from build123d import *

# Parameters (mm, degrees)
SKETCH1_W               = 45
SKETCH1_H               = 67.7
BOSS_EXTRUDE1_DEPTH     = 1.5
CUT_EXTRUDE1_DEPTH      = 41.67336352
CUT_EXTRUDE1_DEPTH_BACK = 41.67336352
SKETCH2_W               = 15
SKETCH2_H               = 3
CUT_EXTRUDE2_DEPTH      = 41.67336352
CUT_EXTRUDE2_DEPTH_BACK = 41.67336352
SKETCH3_R               = 1.5
CUT_EXTRUDE3_DEPTH      = 41.67336352
CUT_EXTRUDE3_DEPTH_BACK = 41.67336352


with BuildPart() as part:
    # Sketch1 → Boss-Extrude1 (new, symmetric)
    with BuildSketch(Plane(origin=(0, 0, 0), x_dir=(1, 0, 0), z_dir=(0, 1, 0))):
        Rectangle(SKETCH1_W, SKETCH1_H)
    extrude(amount=BOSS_EXTRUDE1_DEPTH, both=True)

    # Sketch2 → Cut-Extrude1 (cut, two sides: drawn at the far end of the back side and taken through both)
    with BuildSketch(Plane(origin=(0, 0, 0), x_dir=(1, 0, 0), z_dir=(0, 1, 0)).offset(-CUT_EXTRUDE1_DEPTH_BACK)):
        with Locations((0, -32.35)):
            Rectangle(SKETCH2_W, SKETCH2_H)
        with Locations((0, 32.35)):
            Rectangle(SKETCH2_W, SKETCH2_H)
    extrude(amount=CUT_EXTRUDE1_DEPTH + CUT_EXTRUDE1_DEPTH_BACK, mode=Mode.SUBTRACT)

    # Sketch3 → Cut-Extrude2 (cut, two sides: drawn at the far end of the back side and taken through both)
    with BuildSketch(Plane(origin=(0, 0, 0), x_dir=(1, 0, 0), z_dir=(0, 1, 0)).offset(-CUT_EXTRUDE2_DEPTH_BACK)):
        with Locations(Location((-6.717514421, -17.217514421, 0), (0, 0, 270))):
            Circle(SKETCH3_R)
        with Locations(Location((-6.717514421, 17.217514421, 0), (0, 0, 90))):
            Circle(SKETCH3_R)
        with BuildLine():
            Line((0.072542026, 12.729181386), (-2.119583462, 14.921306874))
            ThreePointArc((-2.119583462, 14.921306874), (-3.083402548, 20.851626294), (-9.013721969, 21.815445381))
            Line((-9.013721969, 21.815445381), (-11.205847457, 24.007570869))
            ThreePointArc((-11.205847457, 24.007570869), (-0.962082205, 22.972946638), (0.072542026, 12.729181386))
        make_face()
        with BuildLine():
            Line((-2.229181386, 10.427457974), (-4.421306874, 12.619583462))
            ThreePointArc((-4.421306874, 12.619583462), (-10.351626294, 13.583402548), (-11.315445381, 19.513721969))
            Line((-11.315445381, 19.513721969), (-13.507570869, 21.705847457))
            ThreePointArc((-13.507570869, 21.705847457), (-12.472946638, 11.462082205), (-2.229181386, 10.427457974))
        make_face()
        with BuildLine():
            Line((0.072542026, -12.729181386), (-2.119583462, -14.921306874))
            ThreePointArc((-2.119583462, -14.921306874), (-3.083402548, -20.851626294), (-9.013721969, -21.815445381))
            Line((-9.013721969, -21.815445381), (-11.205847457, -24.007570869))
            ThreePointArc((-11.205847457, -24.007570869), (-0.962082205, -22.972946638), (0.072542026, -12.729181386))
        make_face()
        with BuildLine():
            Line((-2.229181386, -10.427457974), (-4.421306874, -12.619583462))
            ThreePointArc((-4.421306874, -12.619583462), (-10.351626294, -13.583402548), (-11.315445381, -19.513721969))
            Line((-11.315445381, -19.513721969), (-13.507570869, -21.705847457))
            ThreePointArc((-13.507570869, -21.705847457), (-12.472946638, -11.462082205), (-2.229181386, -10.427457974))
        make_face()
    extrude(amount=CUT_EXTRUDE2_DEPTH + CUT_EXTRUDE2_DEPTH_BACK, mode=Mode.SUBTRACT)

    # Sketch4 → Cut-Extrude3 (cut, two sides: drawn at the far end of the back side and taken through both)
    with BuildSketch(Plane(origin=(0, 0, 0), x_dir=(1, 0, 0), z_dir=(0, 1, 0)).offset(-CUT_EXTRUDE3_DEPTH_BACK)):
        Polygon((-19.5, 0), (-17.25, -1.299038106), (-17.25, 1.299038106), align=None)
    extrude(amount=CUT_EXTRUDE3_DEPTH + CUT_EXTRUDE3_DEPTH_BACK, mode=Mode.SUBTRACT)


solid = part.part
Check sheet for the modelled part. Datum: model origin and axes. Units: mm. A direction names the side the tool comes from. Coordinates: 2 decimals unless noted, no trailing zeros. Write each loop counter-clockwise with the first axis right and the second up, starting at its lowest first coordinate (ties: lowest second). Pieces come first, ordered by that corner, then holes. Notation, with made-up numbers: M 1.25,8.25 L 45.25,8.25 A7 cw 45.25,21.25 Z; hole C 54.25,-13.5 d9. An arc over 180 degrees is marked long. Answer as CSV lines item,"result".
Q1. Cross-section at C-C (z = 20.5). Record the boundary of the cut face in (x, y).
Check result:
outline,"M -22.5,-1.5 L -14.17,-1.5 L -14.17,1.5 L -22.5,1.5 Z; M -12.3,-1.5 L -2.76,-1.5 L -2.76,1.5 L -12.3,1.5 Z; M 0.73,-1.5 L 22.5,-1.5 L 22.5,1.5 L 0.73,1.5 Z"
Q2. Cross-section at D-D (x = -6). Record the boundary of the cut face in (y, z).
Check result:
outline,"M -1.5,-30.85 L 1.5,-30.85 L 1.5,-25.33 L -1.5,-25.33 Z; M -1.5,-22.31 L 1.5,-22.31 L 1.5,-18.53 L -1.5,-18.53 Z; M -1.5,-15.9 L 1.5,-15.9 L 1.5,-12.13 L -1.5,-12.13 Z; M -1.5,-9.11 L 1.5,-9.11 L 1.5,9.11 L -1.5,9.11 Z; M -1.5,12.13 L 1.5,12.13 L 1.5,15.9 L -1.5,15.9 Z; M -1.5,18.53 L 1.5,18.53 L 1.5,22.31 L -1.5,22.31 Z; M -1.5,25.33 L 1.5,25.33 L 1.5,30.85 L -1.5,30.85 Z"
Q3. Go/stop test with a flat-tipped pin: pin 1 (5 mm diameter, centred on x = -6.72, z = -17.22, fed in from -Y). Record where the tip stops, or that it passes through.
Check result:
pin 1,"y = -1.5"
Q4. Cross-section at A-A (x = -18). Record the boundary of the cut face in (y, z), then the cut area to 3 significant figures.
Check result:
outline,"M -1.5,-33.85 L 1.5,-33.85 L 1.5,-0.87 L -1.5,-0.87 Z; M -1.5,0.87 L 1.5,0.87 L 1.5,33.85 L -1.5,33.85 Z"
area,"198 mm^2"
Q5. Cross-section at B-B (y = 0.1). Count the separate pieces of the cut face and the enclosed holes in it, then the cut area to 3 significant figures.
Check result:
separate pieces,"1"
enclosed holes,"7"
area,"2,730 mm^2"
Q6. Mould release check, pull along X, two halves, no side actions. Record for faces 5 (the face through (-12.58, -0.02, 11.57)), 6 (the face through (-15, 0, 33.85)): released by +X, released by -X, zero draft, split by the parting line, or undercut.
Check result:
face 5,"undercut"
face 6,"zero draft"
Q7. Set-up check for faces 1 (the face through (7.5, 0, -32)), 2 (the face through (0, 1.5, 0)), 3 (the face through (-7.5, 0, 32)), 4 (the face through (-1, 0, -13.8)): record each of +Z, -Z, +X, -X, +Y, -Y from which the full face is reachable in a straight line by a thin tool's end or side.
Check result:
face 1,"-Z, +Y, -Y"
face 2,"+Z, -Z, +X, -X, +Y"
face 3,"+Z, +Y, -Y"
face 4,"+Y, -Y"
Q8. Material ranges on probe 1 along Z at (x, y) = (-13.5, 0); probe 2 along Z at (x, y) = (-9, 0.1); probe 3 along Z at (x, y) = (-9.5, 1.2), recorded low to high. Write a range as from..to.
Check result:
probe 1,"-33.85..-21.7, -12.72..12.72, 21.7..33.85"
probe 2,"-33.85..-25.03, -21.82..-12.61, -9.4..9.4, 12.61..21.82, 25.03..33.85"
probe 3,"-33.85..-24.87, -22.3..-12.9, -9.57..9.57, 12.9..22.3, 24.87..33.85"
